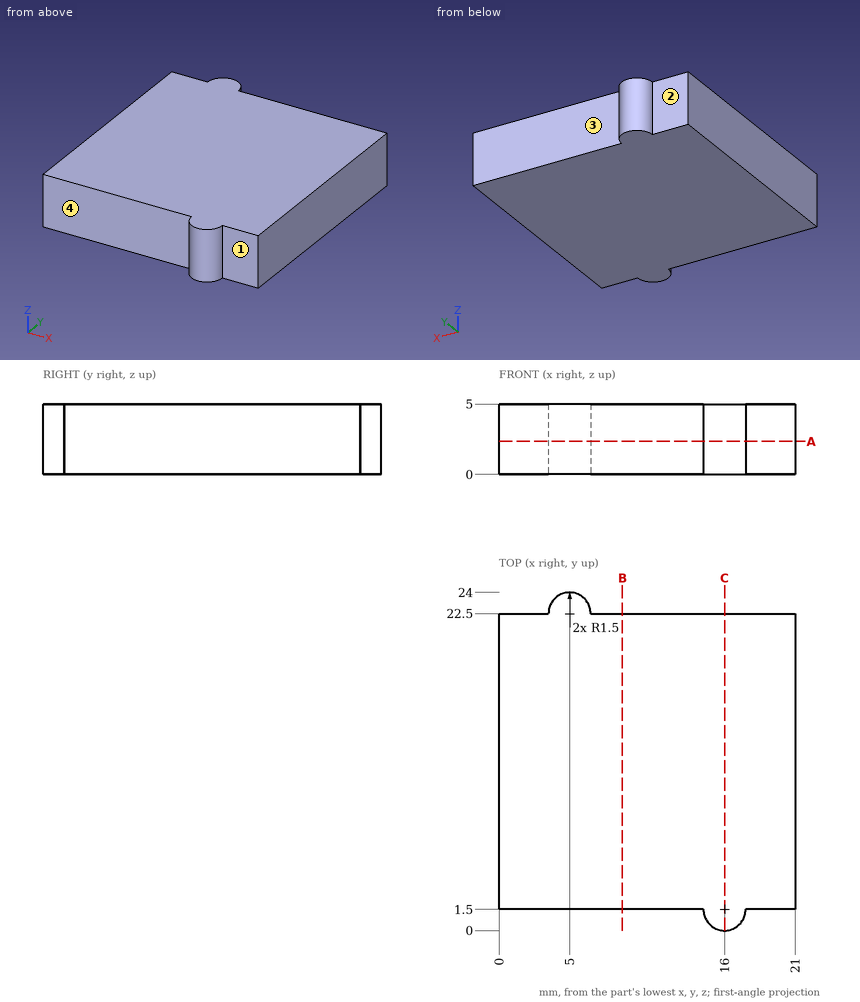
Job drawing, mm, ordinate dimensions from the low corner. One solid piece. A direction names the side the tool comes from. Give positions to 0.01 mm unless a question says otherwise; leave off trailing zeros. Order: outer loops, then holes, each group sorted by start corner. A loop starts at its lowest first (then second) coordinate and runs counter-clockwise, first axis right, second up. Notation, with made-up numbers: (75.5, 61.25) - (120.5, 61.25) arc R22 ccw to (120.5, 78.25) - close; hole circle Ø9 at (8, 27). An arc over 180 degrees is marked (long way). One line per question, with ' | ' between items.
1. Drill centre lines: probe 1 along Y at (x, z) = (7.25, 3.45); probe 2 along Y at (x, z) = (5, 3.4). Where is each one in solid material? Low to high.
Filled in:
probe 1: 1.5 to 22.5 | probe 2: 1.5 to 24
2. Which spindle directions (+Z, -Z, +X, -X, +Y, -Y) get a long thin tool onto all of the face, cutting with end or side? Do the marked faces 1, 2, 3 and 4. Say none if no direction does.
Filled in:
face 1: +Z, -Z, +X, -Y | face 2: +Z, -Z, -X, +Y | face 3: +Z, -Z, +X, +Y | face 4: +Z, -Z, -X, -Y
3. Band-saw the part on A-A on z = 2.35. List the corners of the cut face in (x, y), then the cut area to 3 significant figures.
Filled in:
outline: (0, 1.5) - (14.5, 1.5) arc R1.5 ccw to (17.5, 1.5) - (21, 1.5) - (21, 22.5) - (6.5, 22.5) arc R1.5 ccw to (3.5, 22.5) - (0, 22.5) - close | area: 448 mm²
4. Drop flat-ended pins along their axis: P1, Ø1.5, axis at x = 8.5, z = 3.5, coming from the -Y side; P2, Ø2.5, axis at x = 12, z = 2, coming from the +Y side; P3, Ø2, axis at x = 14, z = 1, coming from the -Y side. Give the stop position or say it passes through.
Filled in:
P1: y = 1.5 | P2: y = 22.5 | P3: y = 0.38
5. Band-saw the part on C-C on x = 16. List the corners of the cut face in (y, z), then the cut area to 4 significant figures.
Filled in:
outline: (0, 0) - (22.5, 0) - (22.5, 5) - (0, 5) - close | area: 112.5 mm²
6. Band-saw the part on B-B on x = 8.75. List the corners of the cut face in (y, z).
Filled in:
outline: (1.5, 0) - (22.5, 0) - (22.5, 5) - (1.5, 5) - close
